from build123d import *

# Parameters (mm, degrees)
BOSS_EXTRU_1_DEPTH      = 11
BOSS_EXTRU_1_DEPTH_BACK = 11
ESQUISSE3_W             = 16.581408451
ESQUISSE3_H             = 12
ENL_V_MAT_EXTRU_2_DEPTH = 40
CUT_EXTRUDE1_REACH      = 158.809
SKETCH1_R               = 1.55
CUT_EXTRUDE2_DEPTH      = 6
FILLET1_R               = 10


with BuildPart() as part:
    # Esquisse1 → Boss.-Extru.1 (new, two sides: drawn at the far end of the back side and taken through both)
    with BuildSketch(Plane.XY.offset(-BOSS_EXTRU_1_DEPTH_BACK)):
        with BuildLine():
            Line((-6.828531952, -151.713036206), (-6.828531952, 91.498065413))
            ThreePointArc((-6.828531952, 91.498065413), (-0.828532479, 94.89251507), (5.171468048, 91.498067278))
            Line((5.171468048, 91.498067278), (5.171468048, -151.713036206))
            ThreePointArc((5.171468048, -151.713036206), (-0.828531952, -155.10748493), (-6.828531952, -151.713036206))
        make_face()
    extrude(amount=BOSS_EXTRU_1_DEPTH + BOSS_EXTRU_1_DEPTH_BACK)

    # Esquisse3 → Enlèv. mat.-Extru.2 (cut)
    with BuildSketch(Plane(origin=(0, 94.89251507, 0), x_dir=(1, 0, 0), z_dir=(0, 1, 0))):
        with Locations((0.202032035, 0)):
            Rectangle(ESQUISSE3_W, ESQUISSE3_H)
    extrude(amount=-ENL_V_MAT_EXTRU_2_DEPTH, mode=Mode.SUBTRACT)

    # Cut-Extrude1: up to this face of the body (flat: up to its plane)
    cut_extrude1_end = Plane(part.part.faces().sort_by_distance((-0.828531947, -30.10748493, -11))[0])
    # Sketch1 → Cut-Extrude1 (cut, up to the picked face)
    with BuildSketch(Plane.XY.offset(11), mode=Mode.PRIVATE) as cut_extrude1_sk1:
        with Locations((-0.828531952, 84.890414662)):
            Circle(SKETCH1_R)
    cut_extrude1_tool1 = split(extrude(cut_extrude1_sk1.sketch, amount=-CUT_EXTRUDE1_REACH, mode=Mode.PRIVATE), bisect_by=cut_extrude1_end, keep=Keep.BOTH, mode=Mode.PRIVATE)
    # Sketch1 → Cut-Extrude1 (cut, up to the picked face)
    with BuildSketch(Plane.XY.offset(11), mode=Mode.PRIVATE) as cut_extrude1_sk2:
        with Locations((-0.828531952, -145.10748493)):
            Circle(SKETCH1_R)
    cut_extrude1_tool2 = split(extrude(cut_extrude1_sk2.sketch, amount=-CUT_EXTRUDE1_REACH, mode=Mode.PRIVATE), bisect_by=cut_extrude1_end, keep=Keep.BOTH, mode=Mode.PRIVATE)
    add(cut_extrude1_tool1.solids().sort_by(Axis((-0.828532, 84.890415, 11), (0, 0, -1)))[0], mode=Mode.SUBTRACT)
    add(cut_extrude1_tool2.solids().sort_by(Axis((-0.828532, -145.107485, 11), (0, 0, -1)))[0], mode=Mode.SUBTRACT)

    # Sketch4 → Cut-Extrude2 (cut)
    with BuildSketch(Plane.XY.offset(11)):
        with BuildLine():
            Line((-6.828531952, 49.278330566), (-6.828531952, -151.713036206))
            ThreePointArc((-6.828531952, -151.713036206), (-0.828531952, -157.713036206), (5.171468048, -151.713036206))
            Line((5.171468048, -151.713036206), (5.171468048, 49.278330566))
            Line((5.171468048, 49.278330566), (-6.828531952, 49.278330566))
        make_face()
    cut_extrude2 = extrude(amount=-CUT_EXTRUDE2_DEPTH, mode=Mode.SUBTRACT)

    # Mirror1: Cut-Extrude2 across plane
    add(cut_extrude2.mirror(Plane.XY), mode=Mode.SUBTRACT)

    # Fillet1
    # the kernel refuses this fillet: 10 mm, written as the material it takes off along each edge
    with BuildSketch(Plane(origin=(28.084346523, 49.278330566, -11), x_dir=(0, 1, 0), z_dir=(-1, 0, 0))) as fillet1_piece_1:
        with BuildLine():
            CenterArc((9.16515139, -10), FILLET1_R, 90, 66.421821522)
            Line((0, -6), (-0.183303028, -5.92))
            ThreePointArc((-0.183303028, -5.92), (-0.2, -3), (-0.2, 0))
            Line((-0.2, 0), (0, 0.2))
            Line((0, 0.2), (9.16515139, 0.2))
            Line((9.16515139, 0.2), (9.16515139, 0))
        make_face()
    extrude(amount=57.82575695, mode=Mode.SUBTRACT)
    with BuildSketch(Plane(origin=(28.084346523, 49.278330566, 11), x_dir=(0, 1, 0), z_dir=(-1, 0, 0))) as fillet1_piece_2:
        with BuildLine():
            CenterArc((9.16515139, 10), FILLET1_R, 203.578178478, 66.421821522)
            Line((0, 6), (-0.183303028, 5.92))
            ThreePointArc((-0.183303028, 5.92), (-0.2, 3), (-0.2, 0))
            Line((-0.2, 0), (0, -0.2))
            Line((0, -0.2), (9.16515139, -0.2))
            Line((9.16515139, -0.2), (9.16515139, 0))
        make_face()
    extrude(amount=57.82575695, mode=Mode.SUBTRACT)


solid = part.part
Input: part model. Units: mm. Frame: model coordinates. A direction names the side the tool comes from. Coordinates: 2 decimals unless noted, no trailing zeros. Order: outer loops, then holes, each group sorted by start corner. A loop starts at its lowest first (then second) coordinate and runs counter-clockwise, first axis right, second up.
1. Contact query for flat-ended pins moving along their axis: P1, Ø1, axis at x = -2.5, z = 7.5, coming from the +Y side; P2, Ø5, axis at x = -4, y = -5.5, coming from the -Z side; P3, Ø4, axis at x = 0, z = -0.5, coming from the -Y side; P4, Ø1.5, axis at x = 1.5, z = -3, coming from the +Y side. Output: stop coordinate, or through.
Checked values:
P1: stops at y = 94.79
P2: stops at z = -5
P3: stops at y = -155.11
P4: stops at y = 54.89
2. Draft query along Z for faces 4 (the flat face through (-1, 54.893, 0)), 5 (the flat face through (-1, 75, -6)), 6 (the flat face through (-1, 77, -11)), 7 (the flat face through (-1, -51, 5)). Return one class per face: +Z half, -Z half, draft (parallel to the pull), parting line (faces both ways), or undercut.
Checked values:
face 4: undercut
face 5: undercut
face 6: -Z half
face 7: +Z half
3. Cut plane C-C, the plane z = 1.5. Return loops of the section in (x, y).
Checked values:
outline: (-6.83, -151.71) arc R7 ccw to (5.17, -151.71) - (5.17, 54.89) - (-6.83, 54.89) - close; hole circle Ø3.1 at (-0.83, -145.11)
4. Cut plane A-A, the plane y = 77. Return loops of the section in (x, z), plus the area to 3 significant figures.
Checked values:
outline: (-6.83, -11) - (5.17, -11) - (5.17, -6) - (-6.83, -6) - close; (-6.83, 6) - (5.17, 6) - (5.17, 11) - (-6.83, 11) - close
area: 120 mm2
5. Cut plane D-D, the plane y = -75.5. Return loops of the section in (x, z), plus the area to 3 significant figures.
Checked values:
outline: (-6.83, -5) - (5.17, -5) - (5.17, 5) - (-6.83, 5) - close
area: 120 mm2
6. Access query for faces 1 (the flat face through (-1, 75, 6)), 2 (the cylindrical face through (-0.93, 94.89, 8.46)), 3 (the flat face through (-1, -51, -5)). Directions: +Z, -Z, +X, -X, +Y, -Y. A direction counts if a zero-diameter tool reaches every point of the face in a straight line with its end or side. Return the directions, or none.
Checked values:
face 1: +X, -X, +Y
face 2: +Z, -Z, +Y
face 3: -Z, +X, -X, -Y
7. Cut plane B-B, the plane x = -4.5. Return loops of the section in (y, z), plus the area to 3 significant figures.
Checked values:
outline: (-154.07, -5) - (49.28, -5) arc R10 ccw to (58.44, -11) - (93.85, -11) - (93.85, -6) - (54.89, -6) - (54.89, 6) - (93.85, 6) - (93.85, 11) - (58.44, 11) arc R10 ccw to (49.28, 5) - (-154.07, 5) - close
area: 2,520 mm2
8. Ray query, line 1 along Z through (x, y) = (2.5, 81); line 2 along Z through (x, y) = (-4.5, -10.5); line 3 along Y through (x, z) = (-1.5, 1.75). Return the intervals inside material, ascending.
Checked values:
line 1: z = -11 to -6, 6 to 11
line 2: z = -5 to 5
line 3: y = -155.08 to -146.5, -143.71 to 54.89
